Geometry check sheet. Reference: the model listing, model coordinates, mm. A direction names the side the tool comes from. Round coordinates to 2 decimals unless told otherwise and drop trailing zeros. Loops run counter-clockwise (first coordinate to the right, second up) from the corner with the lowest first, then second, coordinate; pieces in that order, holes last. Notation, with made-up numbers: (-28, -3.75) - (24, -3.75) arc R29 ccw to (24, 16.25) - close; hole circle Ø5 at (54.5, 38.25). An arc over 180 degrees is marked (long way). Write item = value, one per line.
```python
from build123d import *

# Parameters (mm, degrees)
F1_DEPTH = 70
F2_T     = -2.5
F3_R     = 1


with BuildPart() as f1:
    # F0 (on Top) → F1 (new body)
    with BuildSketch(Plane.XY):
        with BuildLine():
            ThreePointArc((20, 18), (19.4142135624, 19.4142135624), (18, 20))
            Line((18, 20), (-18, 20))
            ThreePointArc((-18, 20), (-19.4142135624, 19.4142135624), (-20, 18))
            Line((-20, 18), (-20, -18))
            ThreePointArc((-20, -18), (-19.4142135624, -19.4142135624), (-18, -20))
            Line((-18, -20), (18, -20))
            ThreePointArc((18, -20), (19.4142135624, -19.4142135624), (20, -18))
            Line((20, -18), (20, 18))
        make_face()
    extrude(amount=F1_DEPTH)

    # F2
    f2_openings = [f1.faces().sort_by_distance(p)[0] for p in [
        (0, 0, 70),
    ]]
    offset(amount=F2_T, openings=f2_openings)

    # F3
    f3_edges = [f1.edges().sort_by_distance(p)[0] for p in [
        (0, -20, 70),
    ]]
    fillet(f3_edges, radius=F3_R)


solid = f1.part
```
(1) Section check A-A (y = 15). Enter the section's corners in (x, z).
Answers follow:
outline = (-20, 0) - (20, 0) - (20, 69) arc R1 ccw to (19, 70) - (17.5, 70) - (17.5, 2.5) - (-17.5, 2.5) - (-17.5, 70) - (-19, 70) arc R1 ccw to (-20, 69) - close
(2) Gauge pin test, flat ends, axial feed: pin 1 (1 mm diameter, centred on x = 7, y = -3.5, fed in from -Z); pin 2 (10.5 mm diameter, centred on x = 8.5, y = -3.5, fed in from +Z). Record the tip position at first contact, or that the pin passes through.
Answers follow:
pin_1 = 0
pin_2 = 2.5
(3) Section check C-C (z = 42.5). Enter the section's corners in (x, y), then the cut area to 3 significant figures.
Answers follow:
outline = (-20, -18) arc R2 ccw to (-18, -20) - (18, -20) arc R2 ccw to (20, -18) - (20, 18) arc R2 ccw to (18, 20) - (-18, 20) arc R2 ccw to (-20, 18) - close; hole (-17.5, -17.5) - (17.5, -17.5) - (17.5, 17.5) - (-17.5, 17.5) - close
area = 372 mm²
(4) Set-up check for faces 1 (the flat face through (-1, -18, 70)), 2 (the flat face through (0, 17.5, 36)): record each of +Z, -Z, +X, -X, +Y, -Y from which the full face is reachable in a straight line by a thin tool's end or side.
Answers follow:
face_1 = +Z, +X, -X, +Y, -Y
face_2 = +Z
(5) Scan lines: L1, parallel to Y at x = 3.5, z = 36; L2, parallel to Z at x = -13, y = 1. Record each from-to range of solid material in increasing order. Write a range as [from, to].
Answers follow:
L1 = [-20, -17.5], [17.5, 20]
L2 = [0, 2.5]
(6) Mould release check, pull along X, two halves, no side actions. Record for faces 3 (the flat face through (-17.5, 0, 36)), 4 (the cylindrical face through (-19.4, 19.43, 34.02)), 5 (the flat face through (0, 0, 0)): pulls with the +X half, pulls with the -X half, needs draft (parallel to the pull), parting line crosses it, or undercut.
Answers follow:
face_3 = undercut
face_4 = pulls with the -X half
face_5 = needs draft
